Geometry: final body of the model. Coordinates: model frame, mm. A direction names the side the tool comes from. Give positions to 0.01 mm unless a question says otherwise; leave off trailing zeros. Write each loop counter-clockwise with the first axis right and the second up, starting at its lowest first coordinate (ties: lowest second). Pieces come first, ordered by that corner, then holes.
Q1. Pin query (flat end, axial travel): pin 1 (1 mm diameter, centred on x = -3.5, y = 8.5, fed in from -Z); pin 2 (12 mm diameter, centred on x = 2, y = 20.5, fed in from +Z); pin 3 (7.5 mm diameter, centred on x = 19, y = 16, fed in from +Z). Return the tip coordinate at first contact, or that it passes through.
Q2. Cut plane C-C on x = 13.5. Return the cut outline in (y, z) (3 decimals).
Q3. Line query: L1, parallel to Z at x = 19.5, y = 3.75 (3 decimals); L2, parallel to X at y = 10.25, z = 6 (3 decimals); L3, parallel to Z at x = -4, y = 10.25. Output: solid intervals per line, ascending.
Q4. Cut plane B-B on z = 18. Return the cut outline in (x, y) (3 decimals), plus the area to 3 significant figures.
Q5. Cut plane A-A on y = 17.75. Return the cut outline in (x, z) (3 decimals).
Q6. Reachability of faces 1 (the face through (21, 13, -19.285)), 2 (the face through (13, 13, -23.095)), 3 (the face through (-24, 13, 0)) from +Z, -Z, +X, -X, +Y, -Y: full face, straight path, thin tool, end or side. Return the list, or none.
Autodesk Fusion 360 part; units mm, degrees
sketch "Sketch1" plane through (0, 0, 0) normal (0, 1, 0) x (1, 0, 0)
  circle A0 centre (0, 0) radius 25 construction
  line L0 (0, -25) -> (0, 25) construction
  line L1 (0, 0) -> (25, 0) construction
  line L2 (0, 0) -> (-25, 0) construction
  line L3 (-25, 0) -> (-23.095, 0)
  line L4 (-23.095, 0) -> (-23.095, -50.8) construction
  line L5 (-23.095, -50.8) -> (-25, -50.8)
  line L6 (-25, -50.8) -> (-25, 0) construction
  line L7 (0, 25) -> (50.8, 25) construction
  line L8 (50.8, 25) -> (50.8, 23.095) construction
  line L9 (50.8, 23.095) -> (0, 23.095) construction
  line L10 (0, 23.095) -> (0, 25)
  line L11 (0, 23.095) -> (25.4, 23.095)
  line L12 (25.4, 23.095) -> (25.4, 19.285)
  line L13 (-23.095, 0) -> (-23.095, -25.4)
  line L14 (-23.095, -25.4) -> (-19.285, -25.4)
  arc A1 (0, 25) -> (-25, 0) centre (0, 0) ccw
  line L15 (-17.6777, 17.6777) -> (0, 0) construction
  line L16 (-19.285, -25.4) -> (-19.285, -15.9088)
  line L17 (25.4, 19.285) -> (15.9088, 19.285)
  arc A2 (15.9088, 19.285) -> (-19.285, -15.9088) centre (16.3882, -16.3882) ccw
  point P0 (-17.6777, 17.6777)
  point P1 (-8.8388, 8.8388)
  dimension "d1" = 50
  dimension "d4" = 50
  dimension "d5" = 1.905
  dimension "d6" = 50.8
  dimension "d7" = 50.8
  dimension "d8" = 1.905
  dimension "d9" = 25.4
  dimension "d10" = 3.81
  dimension "d11" = 25.4
  dimension "d12" = 3.81
  dimension "d13" = 25
  dimension "d15" = 35.6764
extrude "Extrude1" add sketch "Sketch1" along normal blind 25.4
Data:
1. pin 1: stops at z = -24.82
1. pin 2: stops at z = -12.89
1. pin 3: stops at z = -19.27
2. outline: (0, -23.095) - (25.4, -23.095) - (25.4, -19.171) - (0, -19.171) - close
3. L1: z = -23.095 to -19.285
3. L2: x = -23.095 to -17.742
3. L3: z = -24.68 to -12.89
4. outline: (-23.095, 0) - (-19.285, 0) - (-19.285, 25.4) - (-23.095, 25.4) - close
4. area: 96.8 mm2
5. outline: (-25, 0) arc R25 ccw to (0, -25) - (0, -23.095) - (25.4, -23.095) - (25.4, -19.285) - (15.909, -19.285) arc R35.676 cw to (-19.285, 15.909) - (-19.285, 25.4) - (-23.095, 25.4) - (-23.095, 0) - close
6. face 1: +Z, +X, +Y, -Y
6. face 2: -Z, +X, +Y, -Y
6. face 3: +Z, -X, +Y, -Y
